Part print with two shaded views. Sizes in mm from the minimum x, y, z corner. Give positions to 0.01 mm unless a question says otherwise; leave off trailing zeros. Order: outer loops, then holes, each group sorted by start corner. A loop starts at its lowest first (then second) coordinate and runs counter-clockwise, first axis right, second up. Notation, with made-up numbers: (42, 28.25) -> (79, 28.25) arc R22 cw to (79, 55.25) -> close; hole circle Ø5 at (5.5, 3.25). An arc over 180 degrees is marked (long way). Answer as CSV lines item,"result".
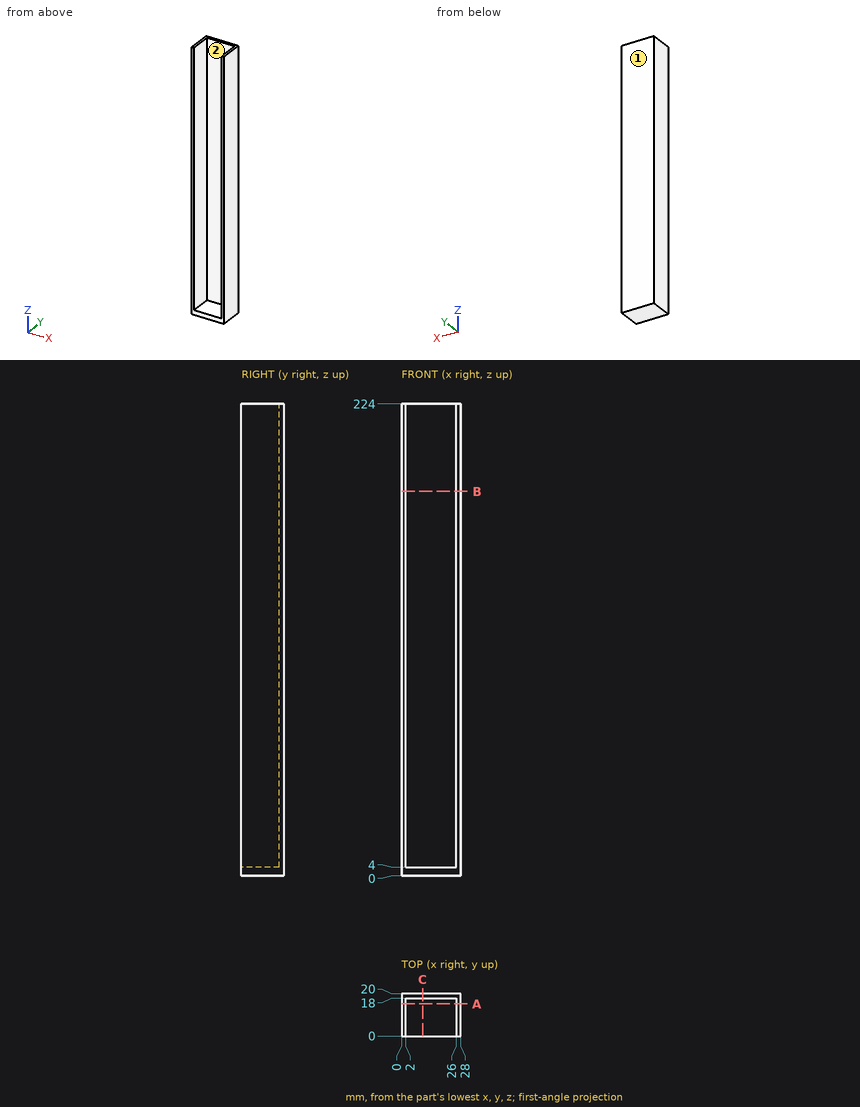
1) Band-saw the part on B-B, the plane z = 182.5. Write the cut outline in (x, y).
Data:
outline,"(0, 0) -> (2, 0) -> (2, 18) -> (26, 18) -> (26, 0) -> (28, 0) -> (28, 20) -> (0, 20) -> close"
2) Pull direction X, two halves, no side cores. Call the marked faces 1 and 2: pulls with the +X half, pulls with the -X half, needs draft (parallel to the pull), parting line crosses it, or undercut.
Data:
face 1,"needs draft"
face 2,"undercut"
3) Wall check: line 1 along X through (y, z) = (16, 174); line 2 along Z through (x, y) = (4, 13); line 3 along Y through (x, z) = (25.25, 79). Give the ranges that are in metal, low to high. Write a range as [from, to].
Data:
line 1,"x = [0, 2], [26, 28]"
line 2,"z = [0, 4]"
line 3,"y = [18, 20]"
4) Pin check, flat tips, straight feed: P1, Ø8, axis at x = 14, y = 6.5, coming from the +Z side; P2, Ø4, axis at y = 12.5, z = 152.5, coming from the -X side. Stop position of each tip, or through.
Data:
P1,"stops at z = 4"
P2,"stops at x = 0"
5) Band-saw the part on C-C, the plane x = 10. Write the cut outline in (y, z), then the cut area to 3 significant figures.
Data:
outline,"(0, 0) -> (20, 0) -> (20, 224) -> (18, 224) -> (18, 4) -> (0, 4) -> close"
area,"520 mm2"
6) Band-saw the part on A-A, the plane y = 15.25. Write the cut outline in (x, z).
Data:
outline,"(0, 0) -> (28, 0) -> (28, 224) -> (26, 224) -> (26, 4) -> (2, 4) -> (2, 224) -> (0, 224) -> close"
